Solid Edge part; units mm, degrees
sketch "Sketch1" plane through (0, 0, 0) normal (0, -1, 0) x (1, 0, 0)
  line L0 (0, 0) -> (40, 0)
  line L1 (40, 0) -> (68.1908, 10.2606)
  line L2 (68.1908, 10.2606) -> (123.1908, 10.2606)
  line L3 (123.1908, 10.2606) -> (123.1908, 16.2606)
  line L4 (123.1908, 16.2606) -> (68.1908, 16.2606)
  line L5 (40, 6) -> (68.1908, 16.2606)
  line L6 (0, 6) -> (40, 6)
  line L7 (0, 0) -> (0, 6)
  dimension "D1" = 123.1908
  dimension "D2" = 123.1908
  dimension "D3" = 40
extrude "Protrusion1" add sketch "Sketch1" along normal blind 20
sketch "Sketch2" plane through (182.9846, -10, 16.2606) normal (0, 0, 1) x (1, 0, 0)
  circle A0 centre (-67.7939, 0) radius 5
  dimension "D1" = 67.7939
extrude "Cutout1" cut sketch "Sketch2" against normal up to surface (6 mm away)
sketch "Sketch3" plane through (43, -10, 6) normal (0, 0, 1) x (1, 0, 0)
  circle A0 centre (-30.8988, 0) radius 0.4991
  circle A1 centre (-30.8988, -0.0009) radius 7.5
  line L0 (-29.3988, 8.4991) -> (-32.3988, 8.4991)
  line L1 (-32.3988, 8.4991) -> (-32.3988, 6.4991)
  line L2 (-32.3988, 6.4991) -> (-29.3988, 6.4991)
  line L3 (-29.3988, 6.4991) -> (-29.3988, 8.4991)
  circle A2 centre (-30.8988, 0) radius 7.5
  dimension "D1" = 32.3988
  dimension "D2" = 32.3988
extrude "Cutout2" cut sketch "Sketch3" against normal up to surface (6 mm away)
Geometry: final body of the model. Coordinates: model frame, mm. A direction names the side the tool comes from. Round coordinates to 2 decimals unless told otherwise and drop trailing zeros. Write each loop counter-clockwise with the first axis right and the second up, starting at its lowest first coordinate (ties: lowest second). Pieces come first, ordered by that corner, then holes. Notation, with made-up numbers: M 20,40.25 L 51,40.25 A18 cw 51,72.25 Z; hole C 12,60.25 d9. An arc over 180 degrees is marked long. Answer in a Markdown table with one row per item. Add a question column.
(1) Cut plane B-B, the plane z = 4. Return the cut outline in (x, y).
(2) Ray query, L1, parallel to Z at x = 29.5, y = -18.5; L2, parallel to Y at x = 6.5, z = 4; L3, parallel to Z at x = 69, y = -4.25. Return the intervals inside material, ascending.
(3) Cut plane A-A, the plane y = -7.5. Return the cut outline in (x, z).
(4) Cut plane C-C, the plane y = -13. Return the cut outline in (x, z).
(5) Contact query for flat-ended pins moving along their axis: pin 1 (2 mm diameter, centred on x = 92.5, z = 12, fed in from +Y); pin 2 (4 mm diameter, centred on x = 46.5, y = -5.5, fed in from +Z); pin 3 (6 mm diameter, centred on x = 104.5, y = -8.5, fed in from -Z). Output: stop coordinate, or through.
(6) Cut plane D-D, the plane x = 71. Return the cut outline in (y, z), then the cut area to 3 significant figures.
(7) Draft query along X for faces 4 (the face through (53.9, -9.86, 5.06)), 5 (the face through (62, -20, 9)), 6 (the face through (12, -1.501, 3)). Return one class per face: pulls with the +X half, pulls with the -X half, needs draft (parallel to the pull), parting line crosses it, or undercut.
(8) Reachability of faces 1 (the face through (62, 0, 9)), 2 (the face through (95, -10, 10.261)), 3 (the face through (24, -10, 6)) from +Z, -Z, +X, -X, +Y, -Y: full face, straight path, thin tool, end or side. Return the list, or none.
Established:
| question | item | result |
|---|---|---|
| 1 | outline | M 0,-20 L 50.99,-20 L 50.99,0 L 0,0 Z; hole M 4.6,-10 A7.5 ccw 19.6,-10 A7.5 ccw 13.6,-2.65 L 13.6,-1.5 L 10.6,-1.5 L 10.6,-2.65 A7.5 ccw Z |
| 2 | L1 | 0 to 6 |
| 2 | L2 | -20 to -14.99, -5.01 to 0 |
| 2 | L3 | 10.26 to 16.26 |
| 3 | outline | M 0,0 L 5.03,0 L 5.03,6 L 0,6 Z; M 19.17,0 L 40,0 L 68.19,10.26 L 110.86,10.26 L 110.86,16.26 L 68.19,16.26 L 40,6 L 19.17,6 Z; M 119.52,10.26 L 123.19,10.26 L 123.19,16.26 L 119.52,16.26 Z |
| 4 | outline | M 0,0 L 5.23,0 L 5.23,6 L 0,6 Z; M 18.98,0 L 40,0 L 68.19,10.26 L 111.19,10.26 L 111.19,16.26 L 68.19,16.26 L 40,6 L 18.98,6 Z; M 119.19,10.26 L 123.19,10.26 L 123.19,16.26 L 119.19,16.26 Z |
| 5 | pin 1 | y = 0 |
| 5 | pin 2 | z = 9.09 |
| 5 | pin 3 | z = 10.26 |
| 6 | outline | M -20,10.26 L 0,10.26 L 0,16.26 L -20,16.26 Z |
| 6 | area | 120 mm² |
| 7 | face 4 | pulls with the +X half |
| 7 | face 5 | needs draft |
| 7 | face 6 | undercut |
| 8 | face 1 | +Z, -Z, +X, -X, +Y |
| 8 | face 2 | -Z, +X, +Y, -Y |
| 8 | face 3 | +Z, -X, +Y, -Y |
